Model file for the job. Use its own axes, mm. A direction names the side the tool comes from. Round coordinates to 2 decimals unless told otherwise and drop trailing zeros. Loops run counter-clockwise (first coordinate to the right, second up) from the corner with the lowest first, then second, coordinate; pieces in that order, holes last. Notation, with made-up numbers: (12, 40) -> (43, 40) arc R26 cw to (43, 73) -> close; hole circle Ø8 at (-2, 55.25). An arc over 180 degrees is marked (long way). Use a Markdown table: item, result.
Autodesk Inventor part; units mm, degrees
ref_plane "YZ Plane" through (0, 0, 0) normal (1, 0, 0) x (0, 1, 0)
ref_plane "XZ Plane" through (0, 0, 0) normal (0, 1, 0) x (-1, 0, 0)
ref_plane "XY Plane" through (0, 0, 0) normal (0, 0, 1) x (1, 0, 0)
sketch "Sketch1" plane through (0, 0, 0) normal (0, 0, 1) x (1, 0, 0)
  line L0 (0, 0) -> (9, 0)
  line L1 (9, 0) -> (9, -5.3835)
  line L2 (9, -5.3835) -> (0, -5.3835)
  line L3 (0, -5.3835) -> (0, 0)
  circle A0 centre (3, -2.2335) radius 1.5
  line L4 (3.4757, -5.3835) -> (9.6132, -5.3835)
  line L5 (9.6132, -5.3835) -> (9.6132, -6.8835)
  line L6 (9.6132, -6.8835) -> (3.4757, -6.8835)
  line L7 (3.4757, -6.8835) -> (3.4757, -5.3835)
  dimension "d0" = 3
  dimension "d1" = 3.15
  dimension "d8" = 1.5
extrude "Extrusion1" add sketch "Sketch1" against normal blind 1.5
extrude "Extrusion2" add sketch "Sketch1" along normal blind 6 and the other way blind 1 contours L4 L5 L6 L7 L2
sketch "Sketch2" plane through (3.4757, -5.3835, 0) normal (0, 1, 0) x (1, 0, 0)
  circle A0 centre (3, -3) radius 1.5
  line L0 (1.0243, 0) -> (-1.9757, 0)
  line L1 (0, 0) -> (0, -6)
  point P0 (-3.4757, 0)
  point P1 (-0.4757, 0)
  dimension "d9" = 3
  dimension "d10" = 3
  dimension "d11" = 3
extrude "Extrusion3" cut sketch "Sketch2" against normal blind 1.5
properties part number "IMU_holder"
Q1. Flat gauge pins, fed straight in: pin 1 (1.2 mm diameter, centred on y = -6.5, z = 1.5, fed in from -X); pin 2 (1 mm diameter, centred on x = 5, z = 3, fed in from -Y); pin 3 (1.6 mm diameter, centred on x = 5.5, y = -2, fed in from +Z); pin 4 (1.2 mm diameter, centred on x = 1.5, z = -0.5, fed in from -Y). Where does each tip first touch, or does it go through?
Results list:
| item | result |
|---|---|
| pin 1 | stops at x = 3.48 |
| pin 2 | stops at y = -6.88 |
| pin 3 | stops at z = 0 |
| pin 4 | stops at y = -5.38 |
Q2. Band-saw the part on D-D, the plane x = 4. Give the cut face in (y, z).
Results list:
| item | result |
|---|---|
| outline | (-6.88, -1.5) -> (-3.35, -1.5) -> (-3.35, 0) -> (-5.38, 0) -> (-5.38, 6) -> (-6.88, 6) -> close; (-1.12, -1.5) -> (0, -1.5) -> (0, 0) -> (-1.12, 0) -> close |
Q3. Band-saw the part on A-A, the plane x = 3. Give the cut face in (y, z).
Results list:
| item | result |
|---|---|
| outline | (-5.38, -1.5) -> (-3.73, -1.5) -> (-3.73, 0) -> (-5.38, 0) -> close; (-0.73, -1.5) -> (0, -1.5) -> (0, 0) -> (-0.73, 0) -> close |
Q4. Band-saw the part on C-C, the plane y = -5.75. Give the cut face in (x, z).
Results list:
| item | result |
|---|---|
| outline | (3.48, -1.5) -> (9.61, -1.5) -> (9.61, 6) -> (3.48, 6) -> close; hole circle Ø3 at (6.48, 3) |
Q5. Pull direction X, two halves, no side cores. Call faces 1 (the face through (5.37, -6.123, 1.986)), 2 (the face through (4.4, -3.3, 0)), 3 (the face through (9.613, -6, 2)): released by +X, released by -X, zero draft, split by the parting line, or undercut.
Results list:
| item | result |
|---|---|
| face 1 | undercut |
| face 2 | zero draft |
| face 3 | released by +X |
Q6. Tool access for faces 4 (the face through (9, -3, -1)), 5 (the face through (2, -5.384, -1)), 6 (the face through (4, 0, -1)): list every direction of +Z, -Z, +X, -X, +Y, -Y with a clear straight run to the whole face (end or side of a thin tool).
Results list:
| item | result |
|---|---|
| face 4 | +Z, -Z, +X, +Y |
| face 5 | +Z, -Z, -X, -Y |
| face 6 | +Z, -Z, +X, -X, +Y |
Q7. Band-saw the part on B-B, the plane z = 3. Give the cut face in (x, y).
Results list:
| item | result |
|---|---|
| outline | (3.48, -6.88) -> (4.98, -6.88) -> (4.98, -5.38) -> (3.48, -5.38) -> close; (7.98, -6.88) -> (9.61, -6.88) -> (9.61, -5.38) -> (7.98, -5.38) -> close |
Q8. Drill centre lines: L1, parallel to Y at x = 3, z = -0.95; L2, parallel to X at y = -6.05, z = 3; L3, parallel to Z at x = 0.5, y = -3.25. Where is each one in solid material? Low to high. Write a range as from..to.
Results list:
| item | result |
|---|---|
| L1 | y = -5.38..-3.73, -0.73..0 |
| L2 | x = 3.48..4.98, 7.98..9.61 |
| L3 | z = -1.5..0 |
